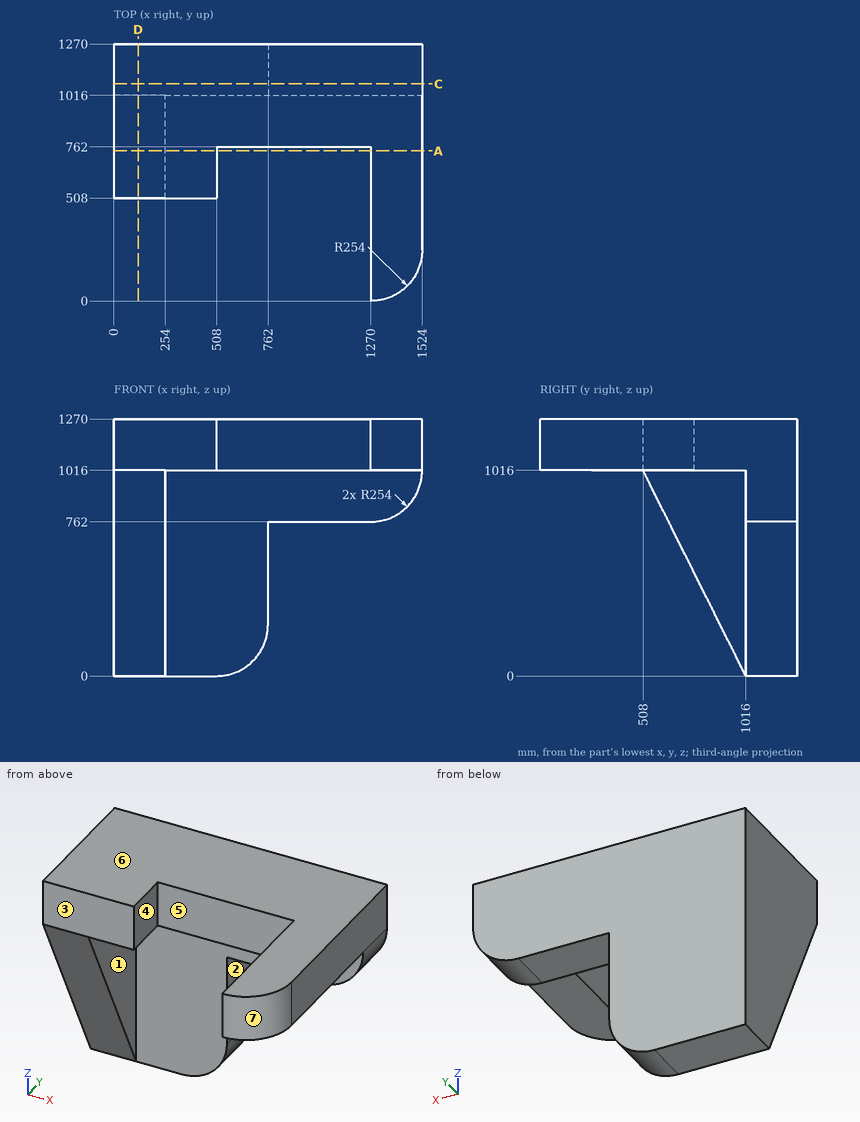
Design review of the part shown in the three views and the two pictorial views. Dimensions are in mm from the part's minimum x, y and z. A direction names the side the tool comes from. Coordinates: 2 decimals unless noted, no trailing zeros. Loops run counter-clockwise (first coordinate to the right, second up) from the corner with the lowest first, then second, coordinate; pieces in that order, holes last.
Q1. We need section D-D on x = 120.5. State the section outline as (y, z) points, and give its area (3 significant figures).
Reported:
outline: (508, 1016) - (1016, 0) - (1270, 0) - (1270, 1270) - (508, 1270) - close
area: 710,000 mm2
Q2. To check wall thickness, follow line 1 (Y direction, x = 594, z = 675); line 2 (X direction, y = 1011.5, z = 297.5). State the ranges of each line that lie inside material, in increasing order.
Reported:
line 1: y = 1016 to 1270
line 2: x = 0 to 254
Q3. We need section A-A on y = 741.5. State the section outline as (x, z) points, and give its area (3 significant figures).
Reported:
outline: (0, 549) - (254, 549) - (254, 1016) - (508, 1016) - (508, 1270) - (0, 1270) - close; (1270, 1016) - (1524, 1016) - (1524, 1270) - (1270, 1270) - close
area: 312,000 mm2
Q4. The part is to be moulded in two halves that separate along X. For the marked faces 5, 6 and 7, say which applies: +X half, -X half, draft (parallel to the pull), parting line (faces both ways), or undercut.
Reported:
face 5: undercut
face 6: draft
face 7: +X half
Q5. We need section C-C on y = 1073. State the section outline as (x, z) points.
Reported:
outline: (0, 0) - (508, 0) arc R254 ccw to (762, 254) - (762, 762) - (1270, 762) arc R254 ccw to (1524, 1016) - (1524, 1270) - (0, 1270) - close
Q6. Tool access review of the marked faces 1, 2, 3 and 4: name each direction out of +Z, -Z, +X, -X, +Y, -Y from which nothing blocks a thin tool from reaching the whole face with its end or side.
Reported:
face 1: -Z, +X, -Y
face 2: -Z, +X, +Y, -Y
face 3: +Z, -Z, -X, -Y
face 4: +Z, -Z, -Y
